Work out the finished part from the listing and answer in its coordinate system (mm). A direction names the side the tool comes from. Give positions to 0.01 mm unless a question says otherwise; leave off trailing zeros. Write each loop counter-clockwise with the first axis right and the second up, starting at its lowest first coordinate (ties: lowest second). Pieces come first, ordered by that corner, then holes. Notation, with made-up numbers: (21.5, 12) -> (51.5, 12) arc R25 ccw to (51.5, 26) -> close; hole circle Ø3 at (50.25, 60). An arc over 180 degrees is marked (long way). Use a Markdown table: item, result. Add a question column.
Q1. Section D-D, the plane y = 15.5 is taken. Give the vertices of the cut face in (x, z).
Q2. Each of these flat-tipped pins is pushed along its axis until it touches: pin 1 Ø0.5 at (x, y) = (31.5, 1.5) entering from +Z; pin 2 Ø3 at (x, y) = (3.5, 21) entering from +Z; pin 3 Ø1.5 at (y, z) = (8, -0.5) entering from -X. Where does it stop, or does it pass through?
Q3. Section C-C, the plane x = 11.5 is taken. Give the vertices of the cut face in (y, z), plus the area to 3 significant figures.
Q4. Consider line 1 (Y direction, x = 0, z = -1.25) (3 decimals); line 2 (Y direction, x = 18, z = 3.5); line 3 (Z direction, x = -3.5, y = 33.5). Determine where each line is inside the solid, lowest interval first.
Q5. For faces 4 (the face through (26.51, 21.38, 0.07)), 5 (the face through (22.85, 22.93, 4.72)), 6 (the face through (21.45, 26.55, 0.07)), determine the directions among +Z, -Z, +X, -X, +Y, -Y from which every point of the face is accessible in a straight line to the end or side of a thin tool.
Q6. Section A-A, the plane y = 0 is taken. Give the vertices of the cut face in (x, z) (3 decimals).
Q7. For a pull along X with two mould halves and no side action, classify faces 1 (the face through (-26.51, -21.38, 0.07)), 2 (the face through (10.866, -26.527, 0.067)), 3 (the face through (25.2, 25.12, -3.58)) as pulls with the +X half, pulls with the -X half, needs draft (parallel to the pull), parting line crosses it, or undercut.
from build123d import *

# Parameters (mm, degrees)
SKETCH1_R           = 31.25
BOSS_EXTRUDE1_DEPTH = 15
BOSS_EXTRUDE2_DEPTH = 4.75
CHAMFER1_SIZE       = 6
CHAMFER1_SIZE2      = 2.183821406
CHAMFER2_SIZE       = 6
CHAMFER2_SIZE2      = 2.183821406
FILLET11_R          = 2
FILLET12_R          = 2
CIRPATTERN1_COUNT   = 8
SKETCH14_W          = 114.781544729
SKETCH14_H          = 99.982125168
CUT_EXTRUDE11_DEPTH = 20
SKETCH15_W          = 194.409122682
SKETCH15_H          = 129.478767366
CUT_EXTRUDE12_DEPTH = 20
CUT_EXTRUDE13_DEPTH = 20
CIRPATTERN3_COUNT   = 8
SKETCH20_R          = 18.625
CUT_EXTRUDE14_DEPTH = 20
SKETCH21_R          = 25
CUT_EXTRUDE15_DEPTH = 2.6


with BuildPart() as part:
    # Sketch1 → Boss-Extrude1 (new body, symmetric)
    with BuildSketch(Plane.XY):
        Circle(SKETCH1_R)
    extrude(amount=BOSS_EXTRUDE1_DEPTH, both=True)

    # Sketch2 → Boss-Extrude2 (add, symmetric)
    with BuildSketch(Plane.XY):
        Polygon((-28.372098708, -5), (-28.372098708, 5), (-38.372098708, 2.5), (-38.372098708, -2.5), align=None)
    extrude(amount=BOSS_EXTRUDE2_DEPTH, both=True)

    # Chamfer1
    chamfer1_edges = [part.edges().sort_by_distance(p)[0] for p in [
        (-38.372098708, 0, -4.75),
    ]]
    chamfer1_side = [part.faces().sort_by_distance(p)[0] for p in [
        (-34.440800156, 0, -4.75),
    ]]
    chamfer(chamfer1_edges, length=CHAMFER1_SIZE, length2=CHAMFER1_SIZE2, reference=chamfer1_side[0])

    # Chamfer2
    chamfer2_edges = [part.edges().sort_by_distance(p)[0] for p in [
        (-38.372098708, 0, 4.75),
    ]]
    chamfer2_side = [part.faces().sort_by_distance(p)[0] for p in [
        (-34.440800156, 0, 4.75),
    ]]
    chamfer(chamfer2_edges, length=CHAMFER2_SIZE, length2=CHAMFER2_SIZE2, reference=chamfer2_side[0])

    # Fillet11
    fillet11_edges = [part.edges().sort_by_distance(p)[0] for p in [
        (-38.372098708, -2.5, 0),
        (-38.372098708, 2.5, 0),
    ]]
    fillet(fillet11_edges, radius=FILLET11_R)

    # Fillet12
    fillet12_edges = [part.edges().sort_by_distance(p)[0] for p in [
        (-32.372098708, 0, -4.75),
        (-32.372098708, 0, 4.75),
    ]]
    fillet(fillet12_edges, radius=FILLET12_R)

    # CirPattern1: part ×8 about axis
    cirpattern1_axis = Axis((0, 0, 0), (0, 0, 1))


with BuildPart() as part_1:
    add(part.part)
    for i in range(1, CIRPATTERN1_COUNT):
        add(part.part.rotate(cirpattern1_axis, i * 360 / CIRPATTERN1_COUNT))

    # Sketch14 → Cut-Extrude11 (cut)
    with BuildSketch(Plane(origin=(0, 0, -4.8), x_dir=(-1, 0, 0), z_dir=(0, 0, -1))):
        with Locations((10.903993862, -9.833989058)):
            Rectangle(SKETCH14_W, SKETCH14_H)
    extrude(amount=CUT_EXTRUDE11_DEPTH, mode=Mode.SUBTRACT)

    # Sketch15 → Cut-Extrude12 (cut)
    with BuildSketch(Plane.XY.offset(4.8)):
        with Locations((1.322307029, -4.255701029)):
            Rectangle(SKETCH15_W, SKETCH15_H)
    extrude(amount=CUT_EXTRUDE12_DEPTH, mode=Mode.SUBTRACT)

    # Sketch17 → Cut-Extrude13 (cut)
    with BuildSketch(Plane.XY.offset(4.8)):
        with BuildLine():
            Line((-3.917153419, 32.703485033), (-4.356824963, 30.944798856))
            ThreePointArc((-4.356824963, 30.944798856), (-10.969884461, 26.483643844), (-18.800536638, 24.962017589))
            Line((-18.800536638, 24.962017589), (-20.35501029, 25.89470178))
            Line((-20.35501029, 25.89470178), (-3.917153419, 32.703485033))
        make_face()
    cut_extrude13 = extrude(amount=-CUT_EXTRUDE13_DEPTH, mode=Mode.SUBTRACT)

    # CirPattern3: Cut-Extrude13 ×8 about axis
    cirpattern3_axis = Axis((0, 0, 0), (0, 0, 1))
    for i in range(1, CIRPATTERN3_COUNT):
        add(cut_extrude13.rotate(cirpattern3_axis, i * 360 / CIRPATTERN3_COUNT), mode=Mode.SUBTRACT)

    # Sketch20 → Cut-Extrude14 (cut)
    with BuildSketch(Plane.XY.offset(4.8)):
        Circle(SKETCH20_R)
    extrude(amount=-CUT_EXTRUDE14_DEPTH, mode=Mode.SUBTRACT)

    # Sketch21 → Cut-Extrude15 (cut)
    with BuildSketch(Plane.XY.offset(4.8)):
        Circle(SKETCH21_R)
    extrude(amount=-CUT_EXTRUDE15_DEPTH, mode=Mode.SUBTRACT)


solid = part_1.part
Result set:
| question | item | result |
|---|---|---|
| 1 | outline | (-25.21, -4.8) -> (-10.33, -4.8) -> (-10.33, 2.2) -> (-19.62, 2.2) -> (-19.62, 4.8) -> (-25.21, 4.8) -> close; (10.33, -4.8) -> (25.21, -4.8) -> (25.21, 4.8) -> (19.62, 4.8) -> (19.62, 2.2) -> (10.33, 2.2) -> close |
| 2 | pin 1 | stops at z = 4.75 |
| 2 | pin 2 | stops at z = 2.2 |
| 2 | pin 3 | stops at x = -28.51 |
| 3 | outline | (-26.27, -4.8) -> (-14.65, -4.8) -> (-14.65, 2.2) -> (-22.2, 2.2) -> (-22.2, 4.8) -> (-26.27, 4.8) -> close; (14.65, -4.8) -> (26.27, -4.8) -> (26.27, 4.8) -> (22.2, 4.8) -> (22.2, 2.2) -> (14.65, 2.2) -> close |
| 3 | area | 184 mm2 |
| 4 | line 1 | y = -38.372 to -18.625, 18.625 to 38.372 |
| 4 | line 2 | y = -24.97 to -17.35, 17.35 to 24.97 |
| 4 | line 3 | z = -4.34 to 4.34 |
| 5 | face 4 | +Z, -Z, +X |
| 5 | face 5 | +Z, +X, +Y |
| 5 | face 6 | +Z, -Z, +Y |
| 6 | outline | (-38.372, -2.566) -> (-32.703, -4.629) arc R2 ccw to (-32.019, -4.75) -> (-31.25, -4.75) -> (-31.25, -4.8) -> (-18.625, -4.8) -> (-18.625, 2.2) -> (-25, 2.2) -> (-25, 4.8) -> (-31.25, 4.8) -> (-31.25, 4.75) -> (-32.019, 4.75) arc R2 ccw to (-32.703, 4.629) -> (-38.372, 2.566) -> close; (18.625, -4.8) -> (31.25, -4.8) -> (31.25, -4.75) -> (32.019, -4.75) arc R2 ccw to (32.703, -4.629) -> (38.372, -2.566) -> (38.372, 2.566) -> (32.703, 4.629) arc R2 ccw to (32.019, 4.75) -> (31.25, 4.75) -> (31.25, 4.8) -> (25, 4.8) -> (25, 2.2) -> (18.625, 2.2) -> close |
| 7 | face 1 | pulls with the -X half |
| 7 | face 2 | undercut |
| 7 | face 3 | pulls with the +X half |
